from build123d import *

# Parameters (mm, degrees)
F0_W     = 19.05
F0_H     = 215.9
F1_DEPTH = 88.9
F2_W     = 203.2
F2_H     = 83.2
F3_DEPTH = 10.16
F4_R     = 2


# Not quite as in the source:
# - a feature names something its author has since deleted; it is built from what else it names


with BuildPart() as f1:
    # F0 (on Top) → F1 (new body)
    with BuildSketch(Plane.XY):
        Rectangle(F0_W, F0_H)
    extrude(amount=F1_DEPTH)

    # F2 (on face) → F3 (cut)
    with BuildSketch(Plane.YZ.offset(9.525)):
        with Locations((0, 41.6)):
            Rectangle(F2_W, F2_H)
    extrude(amount=-F3_DEPTH, mode=Mode.SUBTRACT)

    # F4
    f4_edges = [f1.edges().sort_by_distance(p)[0] for p in [
        (-9.525, 0, 88.9),
        (0, -107.95, 88.9),
        (-9.525, -107.95, 44.45),
        (-9.525, 107.95, 44.45),
        (0, 107.95, 88.9),
        (9.525, 0, 88.9),
        (9.525, -107.95, 44.45),
        (9.525, 107.95, 44.45),
        (-9.525, 0, 0),
        (0, 107.95, 0),
        (0, -107.95, 0),
    ]]
    fillet(f4_edges, radius=F4_R)


solid = f1.part
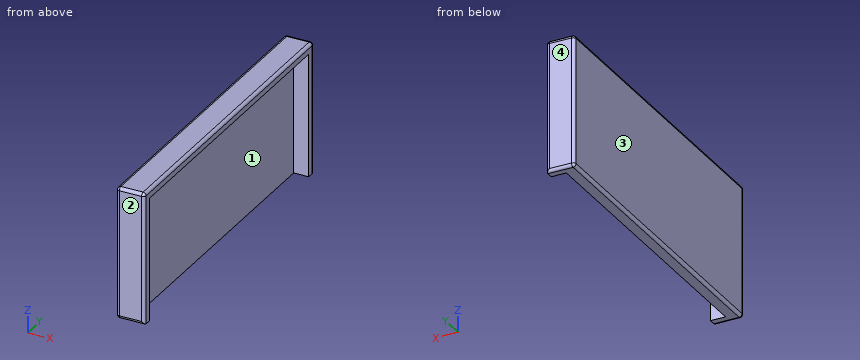
Geometry: final body of the model. Coordinates: model frame, mm. Face numbers are marked on the shaded views. Round coordinates to 2 decimals unless told otherwise and drop trailing zeros. Loops run counter-clockwise (first coordinate to the right, second up) from the corner with the lowest first, then second, coordinate; pieces in that order, holes last. Notation, with made-up numbers: M 7,54 L 63,54 A15 ccw 63,67 Z; hole C 72,58 d10. An arc over 180 degrees is marked long. One line per question, with ' | ' between items.
(1) Cut plane B-B on y = -32.5. Return the cut outline in (x, z) (3 decimals), plus the area to 3 significant figures.
Check result:
outline: M -9.525,2 A2 ccw -7.525,0 L -0.635,0 L -0.635,83.2 L 9.525,83.2 L 9.525,86.9 A2 ccw 7.525,88.9 L -7.525,88.9 A2 ccw -9.525,86.9 Z | area: 846 mm2
(2) Pull-direction query (Y, two-part tool) for the marked faces 1, 2, 3 and 4; classes: +Y half, -Y half, draft (parallel to the pull), parting line (faces both ways), or undercut.
Check result:
face 1: undercut | face 2: -Y half | face 3: draft | face 4: +Y half
(3) Contact query for a flat-ended pin moving along its axis: P1, Ø1.5, axis at y = 75.5, z = 63.5, coming from the +X side (3 decimals). Output: stop coordinate, or through.
Check result:
P1: stops at x = -0.635
(4) Cut plane C-C on z = 63. Return the cut outline in (x, y) (3 decimals).
Check result:
outline: M -9.525,-105.95 A2 ccw -7.525,-107.95 L 7.525,-107.95 A2 ccw 9.525,-105.95 L 9.525,-101.6 L -0.635,-101.6 L -0.635,101.6 L 9.525,101.6 L 9.525,105.95 A2 ccw 7.525,107.95 L -7.525,107.95 A2 ccw -9.525,105.95 Z
(5) Cut plane A-A on x = 2.25. Return the cut outline in (y, z), plus the area to 3 significant figures.
Check result:
outline: M -107.95,2 A2 ccw -105.95,0 L -101.6,0 L -101.6,83.2 L 101.6,83.2 L 101.6,0 L 105.95,0 A2 ccw 107.95,2 L 107.95,86.9 A2 ccw 105.95,88.9 L -105.95,88.9 A2 ccw -107.95,86.9 Z | area: 2,280 mm2
(6) Material intervals for line 1 along Y through (x, z) = (2, 24); line 2 along X through (y, z) = (27.5, 34) (3 decimals); line 3 along Z through (x, y) = (2.25, -22.5), sorted ascending. Write a range as from..to.
Check result:
line 1: y = -107.95..-101.6, 101.6..107.95 | line 2: x = -9.525..-0.635 | line 3: z = 83.2..88.9
